from build123d import *

# Parameters (mm, degrees)
F1_DEPTH = 10
F2_R     = 20
F3_DEPTH = 20
F0_W     = 25
F0_H     = 10
F4_DEPTH = 5
F5_R     = 8


with BuildPart() as f1:
    # F0 (on Top) → F1 (new body)
    with BuildSketch(Plane.XY):
        with BuildLine():
            Line((0, 10), (-36.8826230851, 10))
            ThreePointArc((-36.8826230851, 10), (-35.4747537924, 5.0878352391), (-35, 0))
            ThreePointArc((-35, 0), (-35.4747537924, -5.0878352391), (-36.8826230851, -10))
            Line((-36.8826230851, -10), (0, -10))
            Line((0, -10), (0, -5))
            Line((0, -5), (-25, -5))
            Line((-25, -5), (-25, 5))
            Line((-25, 5), (0, 5))
            Line((0, 5), (0, 10))
        make_face()
        with BuildLine():
            Line((-114.3075854453, 51.8075854453), (-81.9454364826, 19.4454364826))
            ThreePointArc((-81.9454364826, 19.4454364826), (-80.0890590993, 21.1394181566), (-78.08578927, 22.6568570819))
            Line((-78.08578927, 22.6568570819), (-112.0176888624, 56.5887566742))
            ThreePointArc((-112.0176888624, 56.5887566742), (-113.1878851609, 54.2102633531), (-114.3075854453, 51.8075854453))
        make_face()
        with BuildLine():
            ThreePointArc((-85.1568570819, 15.58578927), (-83.6394181566, 17.5890590993), (-81.9454364826, 19.4454364826))
            Line((-81.9454364826, 19.4454364826), (-114.3075854453, 51.8075854453))
            ThreePointArc((-114.3075854453, 51.8075854453), (-115.3931446982, 49.3423971515), (-116.4255463439, 46.8544785321))
            Line((-116.4255463439, 46.8544785321), (-85.1568570819, 15.58578927))
        make_face()
        with BuildLine():
            ThreePointArc((-78.4099025767, 15.9099025767), (-53.8896227718, 20.7872894815), (-40, 0))
            ThreePointArc((-40, 0), (-53.8896227718, -20.7872894815), (-78.4099025767, -15.9099025767))
            Line((-78.4099025767, -15.9099025767), (-81.9454364826, -19.4454364826))
            ThreePointArc((-81.9454364826, -19.4454364826), (-80.0890590993, -21.1394181566), (-78.08578927, -22.6568570819))
            ThreePointArc((-78.08578927, -22.6568570819), (-54.424902758, -26.2876930242), (-36.8826230851, -10))
            ThreePointArc((-36.8826230851, -10), (-35.4747537924, -5.0878352391), (-35, 0))
            ThreePointArc((-35, 0), (-35.4747537924, 5.0878352391), (-36.8826230851, 10))
            ThreePointArc((-36.8826230851, 10), (-54.424902758, 26.2876930242), (-78.08578927, 22.6568570819))
            ThreePointArc((-78.08578927, 22.6568570819), (-80.0890590993, 21.1394181566), (-81.9454364826, 19.4454364826))
            Line((-81.9454364826, 19.4454364826), (-78.4099025767, 15.9099025767))
        make_face()
        with BuildLine():
            ThreePointArc((-78.4099025767, -15.9099025767), (-85, 0), (-78.4099025767, 15.9099025767))
            Line((-78.4099025767, 15.9099025767), (-81.9454364826, 19.4454364826))
            ThreePointArc((-81.9454364826, 19.4454364826), (-83.6394181566, 17.5890590993), (-85.1568570819, 15.58578927))
            ThreePointArc((-85.1568570819, 15.58578927), (-90, 0), (-85.1568570819, -15.58578927))
            ThreePointArc((-85.1568570819, -15.58578927), (-83.6394181566, -17.5890590993), (-81.9454364826, -19.4454364826))
            Line((-81.9454364826, -19.4454364826), (-78.4099025767, -15.9099025767))
        make_face()
        with BuildLine():
            Line((-114.3075854453, -51.8075854453), (-81.9454364826, -19.4454364826))
            ThreePointArc((-81.9454364826, -19.4454364826), (-83.6394181566, -17.5890590993), (-85.1568570819, -15.58578927))
            Line((-85.1568570819, -15.58578927), (-116.4255463439, -46.8544785321))
            ThreePointArc((-116.4255463439, -46.8544785321), (-115.3931446982, -49.3423971515), (-114.3075854453, -51.8075854453))
        make_face()
        with BuildLine():
            ThreePointArc((-78.08578927, -22.6568570819), (-80.0890590993, -21.1394181566), (-81.9454364826, -19.4454364826))
            Line((-81.9454364826, -19.4454364826), (-114.3075854453, -51.8075854453))
            ThreePointArc((-114.3075854453, -51.8075854453), (-113.1878851609, -54.2102633531), (-112.0176888624, -56.5887566742))
            Line((-112.0176888624, -56.5887566742), (-78.08578927, -22.6568570819))
        make_face()
        with BuildLine():
            ThreePointArc((-112.0176888624, -56.5887566742), (-113.1878851609, -54.2102633531), (-114.3075854453, -51.8075854453))
            ThreePointArc((-114.3075854453, -51.8075854453), (-115.3931446982, -49.3423971515), (-116.4255463439, -46.8544785321))
            Line((-116.4255463439, -46.8544785321), (-122.731528021, -53.1604602091))
            ThreePointArc((-122.731528021, -53.1604602091), (-120.5294282278, -57.98033659), (-118.1381334557, -62.7092012675))
            Line((-118.1381334557, -62.7092012675), (-112.0176888624, -56.5887566742))
        make_face()
        with BuildLine():
            ThreePointArc((-116.4255463439, 46.8544785321), (-115.3931446982, 49.3423971515), (-114.3075854453, 51.8075854453))
            ThreePointArc((-114.3075854453, 51.8075854453), (-113.1878851609, 54.2102633531), (-112.0176888624, 56.5887566742))
            Line((-112.0176888624, 56.5887566742), (-118.1381334557, 62.7092012675))
            ThreePointArc((-118.1381334557, 62.7092012675), (-120.5294282278, 57.98033659), (-122.731528021, 53.1604602091))
            Line((-122.731528021, 53.1604602091), (-116.4255463439, 46.8544785321))
        make_face()
    extrude(amount=F1_DEPTH)

    # F2
    f2_edges = [f1.edges().sort_by_distance(p)[0] for p in [
        (-78.085789, -22.656857, 5),
        (-36.882623, -10, 5),
        (-36.882623, 10, 5),
        (-78.085789, 22.656857, 5),
        (-85.156857, -15.585789, 5),
        (-85.156857, 15.585789, 5),
    ]]
    fillet(f2_edges, radius=F2_R)

    # F0 (on Top) → F3 (join)
    with BuildSketch(Plane.XY):
        with BuildLine():
            ThreePointArc((-116.4255463439, 46.8544785321), (-115.3931446982, 49.3423971515), (-114.3075854453, 51.8075854453))
            ThreePointArc((-114.3075854453, 51.8075854453), (-113.1878851609, 54.2102633531), (-112.0176888624, 56.5887566742))
            Line((-112.0176888624, 56.5887566742), (-118.1381334557, 62.7092012675))
            ThreePointArc((-118.1381334557, 62.7092012675), (-120.5294282278, 57.98033659), (-122.731528021, 53.1604602091))
            Line((-122.731528021, 53.1604602091), (-116.4255463439, 46.8544785321))
        make_face()
        with BuildLine():
            ThreePointArc((-112.0176888624, -56.5887566742), (-113.1878851609, -54.2102633531), (-114.3075854453, -51.8075854453))
            ThreePointArc((-114.3075854453, -51.8075854453), (-115.3931446982, -49.3423971515), (-116.4255463439, -46.8544785321))
            Line((-116.4255463439, -46.8544785321), (-122.731528021, -53.1604602091))
            ThreePointArc((-122.731528021, -53.1604602091), (-120.5294282278, -57.98033659), (-118.1381334557, -62.7092012675))
            Line((-118.1381334557, -62.7092012675), (-112.0176888624, -56.5887566742))
        make_face()
    extrude(amount=F3_DEPTH)

    # F0 (on Top) → F4 (join)
    with BuildSketch(Plane.XY):
        with Locations((-12.5, 0)):
            Rectangle(F0_W, F0_H)
    extrude(amount=F4_DEPTH)

    # F5
    f5_edges = [f1.edges().sort_by_distance(p)[0] for p in [
        (-120.529428, -57.980337, 20),
        (-120.529428, 57.980337, 20),
    ]]
    fillet(f5_edges, radius=F5_R)


solid = f1.part
Geometry check sheet. Reference: the model listing, model coordinates, mm. A direction names the side the tool comes from. Give positions to 0.01 mm unless a question says otherwise; leave off trailing zeros. Loops run counter-clockwise (first coordinate to the right, second up) from the corner with the lowest first, then second, coordinate; pieces in that order, holes last. Notation, with made-up numbers: (45, 57) -> (101, 57) arc R16 cw to (101, 79) -> close; hole circle Ø6 at (-33.75, -25). An arc over 180 degrees is marked (long way). Answer in a Markdown table with one row per item. Add a question column.
1) Gauge pin test, flat ends, axial feed: P1, Ø2.5, axis at y = 0.5, z = 8.5, coming from the +X side; P2, Ø5.5, axis at x = -11.5, z = 8, coming from the -Y side; P3, Ø2.5, axis at x = -16.5, z = 7.5, coming from the +Y side; P4, Ø2, axis at x = -32.5, y = -7, coming from the -Z side. Record the tip position at first contact, or that the pin passes through.
2) Draft check along Y on faces 4 (the face through (0, 0, 4)), 5 (the face through (-53.436, 25.963, 4.93)), 6 (the face through (-13, 5, 7)), 7 (the face through (-12, -5, 7)). Enter one of: pulls with the +Y half, pulls with the -Y half, needs draft (parallel to the pull), parting line crosses it, or undercut.
3) Cross-section at C-C on z = 2. Record the boundary of the cut face in (x, y).
4) Material ranges on probe 1 along Y at (x, z) = (-115, 9.75); probe 2 along X at (y, z) = (4, 9.25); probe 3 along Y at (x, z) = (-108.5, 8.5), recorded low to high. Write a range as from..to.
5) Cross-section at D-D on x = -104. Record the boundary of the cut face in (y, z), and give its area (3 significant figures).
6) Set-up check for faces 1 (the face through (-120.497, 58.047, 5.916)), 2 (the face through (-25, 0, 7)), 3 (the face through (-13, 10, 5)): record each of +Z, -Z, +X, -X, +Y, -Y from which the full face is reachable in a straight line by a thin tool's end or side.
7) Cross-section at B-B on z = 14. Record the boundary of the cut face in (x, y).
8) Cross-section at A-A on x = -80. Record the boundary of the cut face in (y, z), and give its area (3 significant figures).
Outcome:
| question | item | result |
|---|---|---|
| 1 | P1 | stops at x = -25 |
| 1 | P2 | stops at y = -10 |
| 1 | P3 | stops at y = 10 |
| 1 | P4 | stops at z = 0 |
| 2 | face 4 | needs draft |
| 2 | face 5 | pulls with the +Y half |
| 2 | face 6 | undercut |
| 2 | face 7 | undercut |
| 3 | outline | (-122.73, -53.16) arc R133.75 ccw to (-118.14, -62.71) -> (-87.52, -32.09) arc R20 cw to (-68.8, -26.77) arc R27.5 ccw to (-41.18, -17.37) arc R20 cw to (-25.67, -10) -> (0, -10) -> (0, 10) -> (-25.67, 10) arc R20 cw to (-41.18, 17.37) arc R27.5 ccw to (-68.8, 26.77) arc R20 cw to (-87.52, 32.09) -> (-118.14, 62.71) arc R133.75 ccw to (-122.73, 53.16) -> (-94.59, 25.02) arc R20 cw to (-89.27, 6.3) arc R27.5 ccw to (-89.27, -6.3) arc R20 cw to (-94.59, -25.02) -> close; hole circle Ø45 at (-62.5, 0) |
| 4 | probe 1 | y = -59.57..-45.43, 45.43..59.57 |
| 4 | probe 2 | x = -89.71..-84.64, -40.36..-25 |
| 4 | probe 3 | y = -53.07..-38.93, 38.93..53.07 |
| 5 | outline | (-48.57, 0) -> (-34.43, 0) -> (-34.43, 10) -> (-48.57, 10) -> close; (34.43, 0) -> (48.57, 0) -> (48.57, 10) -> (34.43, 10) -> close |
| 5 | area | 283 mm^2 |
| 6 | face 1 | +Z, -Z, -X, +Y |
| 6 | face 2 | +Z, +X |
| 6 | face 3 | +Z, -Z, +X, +Y |
| 7 | outline | (-122.54, -52.97) arc R133.5 ccw to (-117.95, -62.52) -> (-112.02, -56.59) arc R125.5 cw to (-116.43, -46.85) -> close; (-122.54, 52.97) -> (-116.43, 46.85) arc R125.5 cw to (-112.02, 56.59) -> (-117.95, 62.52) arc R133.5 ccw to start |
| 8 | outline | (-27.36, 0) -> (-14.14, 0) -> (-14.14, 10) -> (-27.36, 10) -> close; (14.14, 0) -> (27.36, 0) -> (27.36, 10) -> (14.14, 10) -> close |
| 8 | area | 264 mm^2 |
